from build123d import *

# Parameters (mm, degrees)
BOSS_EXTRUDE1_DEPTH = 12
SKETCH2_R           = 4.75
BOSS_EXTRUDE2_DEPTH = 61
CUT_EXTRUDE1_DEPTH  = 14


with BuildPart() as part:
    # Sketch1 → Boss-Extrude1 (new body)
    with BuildSketch(Plane.XY):
        Polygon((3.666174209, -6.35), (7.332348419, 0), (3.666174209, 6.35), (-3.666174209, 6.35), (-7.332348419, 0), (-3.666174209, -6.35), align=None)
    extrude(amount=BOSS_EXTRUDE1_DEPTH)

    # Sketch2 → Boss-Extrude2 (add)
    with BuildSketch(Plane(origin=(0, 0, 0), x_dir=(-1, 0, 0), z_dir=(0, 0, -1))):
        with Locations(Location((0, 0, 0), (0, 0, 180))):
            Circle(SKETCH2_R)
    extrude(amount=BOSS_EXTRUDE2_DEPTH)

    # Sketch3 → Cut-Extrude1 (cut)
    with BuildSketch(Plane(origin=(0, 0, -61), x_dir=(-1, 0, 0), z_dir=(0, 0, -1))):
        with BuildLine():
            Line((-2.645751311, 3), (2.645751311, 3))
            ThreePointArc((2.645751311, 3), (4, 0), (2.645751311, -3))
            Line((2.645751311, -3), (-2.645751311, -3))
            ThreePointArc((-2.645751311, -3), (-4, 0), (-2.645751311, 3))
        make_face()
    extrude(amount=-CUT_EXTRUDE1_DEPTH, mode=Mode.SUBTRACT)


solid = part.part
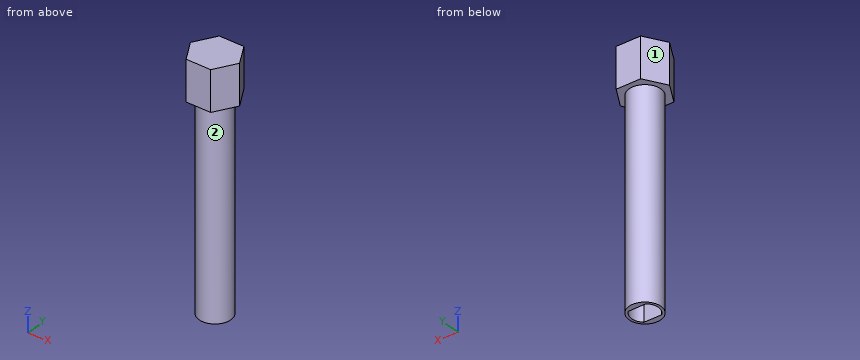
Source: CAD feature listing. Evaluate the final solid. Frame: model axes, mm. Face numbers are marked on the shaded views. A direction names the side the tool comes from. Coordinates: 2 decimals unless noted, no trailing zeros. Loops run counter-clockwise (first coordinate to the right, second up) from the corner with the lowest first, then second, coordinate; pieces in that order, holes last. Notation, with made-up numbers: (32, 64.25) - (60, 64.25) arc R26 cw to (60, 79.25) - close; hole circle Ø1 at (30, 65.5). An arc over 180 degrees is marked (long way). Return JSON: item names as keys, results as strings.
Q1. Material intervals for line 1 along Z through (x, y) = (2.5, -1.5); line 2 along Y through (x, z) = (2, -39); line 3 along X through (y, z) = (3, 6.5), sorted ascending.
Results:
{"line 1": "-47 to 12", "line 2": "-4.31 to 4.31", "line 3": "-5.6 to 5.6"}
Q2. Section B-B, the plane x = 0. Return loops of the section in (y, z), plus the area to 3 significant figures.
Results:
{"outline": "(-6.35, 0) - (-4.75, 0) - (-4.75, -61) - (-3, -61) - (-3, -47) - (3, -47) - (3, -61) - (4.75, -61) - (4.75, 0) - (6.35, 0) - (6.35, 12) - (-6.35, 12) - close", "area": "648 mm2"}
Q3. Access query for the marked faces 1 and 2. Directions: +Z, -Z, +X, -X, +Y, -Y. A direction counts if a zero-diameter tool reaches every point of the face in a straight line with its end or side. Return the directions, or none.
Results:
{"face 1": "+Z, -Z, -X, +Y", "face 2": "-Z"}
Q4. Section A-A, the plane z = -51. Return loops of the section in (x, y), plus the area to 3 significant figures.
Results:
{"outline": "circle Ø9.5 at (0, 0); hole (-2.65, -3) - (2.65, -3) arc R4 ccw to (2.65, 3) - (-2.65, 3) arc R4 ccw to start", "area": "27.9 mm2"}
Q5. Contact query for flat-ended pins moving along their axis: P1, Ø6, axis at x = -1, z = -52, coming from the -Y side; P2, Ø1, axis at y = 0.5, z = -4, coming from the -X side; P3, Ø3, axis at x = 0.5, y = 0, coming from the -Z side. Output: stop coordinate, or through.
Results:
{"P1": "y = -4.75", "P2": "x = -4.75", "P3": "z = -47"}
Q6. Section C-C, the plane y = 1.75. Return loops of the section in (x, z).
Results:
{"outline": "(-6.32, 0) - (-4.42, 0) - (-4.42, -61) - (-3.6, -61) - (-3.6, -47) - (3.6, -47) - (3.6, -61) - (4.42, -61) - (4.42, 0) - (6.32, 0) - (6.32, 12) - (-6.32, 12) - close"}
Q7. Section D-D, the plane z = -13. Return loops of the section in (x, y).
Results:
{"outline": "circle Ø9.5 at (0, 0)"}
